from build123d import *

# Parameters (mm, degrees)
SKETCH1_W           = 127
SKETCH1_H           = 12.7
BOSS_EXTRUDE1_DEPTH = 3.175
FILLET1_R           = 6.35
SKETCH2_R           = 3.175
SKETCH2_R_2         = 1.905
CUT_EXTRUDE1_DEPTH  = 3.175
FILLET2_R           = 6.35


with BuildPart() as part:
    # Sketch1 → Boss-Extrude1 (new body)
    with BuildSketch(Plane.XY):
        with Locations((63.5, 6.35)):
            Rectangle(SKETCH1_W, SKETCH1_H)
    extrude(amount=BOSS_EXTRUDE1_DEPTH)

    # Fillet1
    fillet1_edges = [part.edges().sort_by_distance(p)[0] for p in [
        (0, 0, 1.5875),
        (0, 12.7, 1.5875),
    ]]
    fillet(fillet1_edges, radius=FILLET1_R - 0.0001)  # a hair under: the kernel refuses the full size

    # Sketch2 → Cut-Extrude1 (cut)
    with BuildSketch(Plane.XY.offset(3.175)):
        with Locations((6.35, 6.35)):
            Circle(SKETCH2_R)
        with Locations((120.396, 6.35)):
            Circle(SKETCH2_R_2)
    extrude(amount=-CUT_EXTRUDE1_DEPTH, mode=Mode.SUBTRACT)

    # Fillet2
    fillet2_edges = [part.edges().sort_by_distance(p)[0] for p in [
        (127, 0, 1.5875),
        (127, 12.7, 1.5875),
    ]]
    fillet(fillet2_edges, radius=FILLET2_R - 0.0001)  # a hair under: the kernel refuses the full size


solid = part.part
Verification items for the finished model (mm, model axes). Coordinates: 2 decimals unless noted, no trailing zeros. Order: outer loops, then holes, each group sorted by start corner. A loop starts at its lowest first (then second) coordinate and runs counter-clockwise, first axis right, second up. Notation, with made-up numbers: M -14,65 L 0,65 A34 cw 0,101 Z; hole C 18,-5 d3. An arc over 180 degrees is marked long. One line per item, written item: value. Start each with the question number.
Item 1: Sectioned sample at A-A on z = 2.6. Give the number of separate pieces and of enclosed holes in the cut face, then the cut area to 3 significant figures.
Item 2: Depth check by flat-ended pin: P1, Ø4, axis at x = 6.35, y = 6.35, coming from the +Z side. Enter the tip coordinate at first touch or a pass-through.
Item 3: Mould release check, pull along Y, two halves, no side actions. Record for faces 1 (the cylindrical face through (122.156, 5.62, 1.61)), 2 (the cylindrical face through (4.01, 8.496, 1.61)), 3 (the flat face through (63, 6, 3.175)), 4 (the cylindrical face through (1.81, 1.91, 1.61)): pulls with the +Y half, pulls with the -Y half, needs draft (parallel to the pull), parting line crosses it, or undercut.
Item 4: Thickness scan on probe 1 along X at (y, z) = (8, 2.75); probe 2 along Y at (x, z) = (6.35, 1.9) (3 decimals); probe 3 along X at (y, z) = (4.75, 1.5). Record the ranges inside material, lowest first.
Item 5: Sectioned sample at B-B on y = 1.25. Record the cut outline in (x, z) (3 decimals).
Calculated:
1. separate pieces: 1
1. enclosed holes: 2
1. area: 1,540 mm^2
2. P1: through
3. face 1: undercut
3. face 2: undercut
3. face 3: needs draft
3. face 4: pulls with the -Y half
4. probe 1: 0.22 to 3.64, 9.06 to 119.44, 121.35 to 126.78
4. probe 2: 0 to 3.175, 9.525 to 12.7
4. probe 3: 0.2 to 3.61, 9.09 to 119.36, 121.43 to 126.8
5. outline: M 2.567,0 L 124.433,0 L 124.433,3.175 L 2.567,3.175 Z
